For this review, take the finished solid that the model builds, in its own axes (mm). Coordinates: 2 decimals unless noted, no trailing zeros. Order: outer loops, then holes, each group sorted by start corner. A loop starts at its lowest first (then second) coordinate and runs counter-clockwise, first axis right, second up. Notation, with made-up numbers: (53.25, 77) -> (86.25, 77) arc R8 ccw to (86.25, 92) -> close; hole circle Ø8 at (8, 80.5). An arc over 180 degrees is marked (long way). Return JSON: item names as keys, results as strings. Group by question number.
Item 1: Take a section at B-B (x = -15). Write out the cut boundary in (y, z).
Item 2: For line 1 along X through (y, z) = (15.15, 10); line 2 along X through (y, z) = (15.2, 55); line 3 along Z through (x, y) = (-11, 14.8), list the stretches that pass through material, from the lowest coordinate up.
Item 3: Insertion check: pin 1 (6 mm diameter, centred on x = -2, z = 52, fed in from +Y); pin 2 (1.6 mm diameter, centred on x = -1.5, y = 11, fed in from +Z); pin 3 (1.5 mm diameter, centred on x = -0.5, z = 31.5, fed in from -Y); pin 4 (2 mm diameter, centred on x = -24, z = 12.5, fed in from -Y). Each pin has a flat end and moves straight along its axis. Give the tip position at first contact, or say it passes through.
Item 4: Take a section at D-D (x = -4). Write out the cut boundary in (y, z).
Item 5: Take a section at C-C (z = 32.5). Write out the cut boundary in (x, y).
Item 6: Take a section at A-A (z = 10). Write out the cut boundary in (x, y).
```python
from build123d import *

# Parameters (mm, degrees)
SKETCH1_W           = 45.5
SKETCH1_H           = 3
BOSS_EXTRUDE1_DEPTH = 20
SKETCH2_W           = 45.5
SKETCH2_H           = 3
BOSS_EXTRUDE2_DEPTH = 45
SKETCH3_R           = 8.25
CUT_EXTRUDE1_DEPTH  = 75.656105932
CUT_EXTRUDE2_DEPTH  = 75.656105932
BOSS_EXTRUDE4_DEPTH = 3
CUT_EXTRUDE3_DEPTH  = 75.656105932
SKETCH10_W          = 10
SKETCH10_H          = 2.5
CUT_EXTRUDE4_DEPTH  = 2
SKETCH13_W          = 3
SKETCH13_H          = 14.133974596
CUT_EXTRUDE6_DEPTH  = 1
CHAMFER1_SIZE       = 1
SKETCH15_R          = 2.25
CUT_EXTRUDE7_DEPTH  = 75.788557826
CHAMFER2_SIZE       = 1


with BuildPart() as part:
    # Sketch1 → Boss-Extrude1 (new body)
    with BuildSketch(Plane.XY):
        with Locations((-13.849646897, 14.534741944)):
            Rectangle(SKETCH1_W, SKETCH1_H)
    extrude(amount=BOSS_EXTRUDE1_DEPTH)

    # Sketch2 → Boss-Extrude2 (add)
    with BuildSketch(Plane.XY.offset(20)):
        with Locations((-13.849646897, 14.534741944)):
            Rectangle(SKETCH2_W, SKETCH2_H)
    extrude(amount=BOSS_EXTRUDE2_DEPTH)

    # Sketch3 → Cut-Extrude1 (cut, through all)
    with BuildSketch(Plane(origin=(0, 13.034741944, 0), x_dir=(-1, 0, 0), z_dir=(0, -1, 0))):
        with Locations(Location((26.924646897, -55, 0), (0, 0, 90))):
            Circle(SKETCH3_R)
        with Locations(Location((0.774646897, -55, 0), (0, 0, 90))):
            Circle(SKETCH3_R)
    extrude(amount=-CUT_EXTRUDE1_DEPTH, mode=Mode.SUBTRACT)

    # Sketch5 → Cut-Extrude2 (cut, through all)
    with BuildSketch(Plane(origin=(0, 13.034741944, 0), x_dir=(-1, 0, 0), z_dir=(0, -1, 0))):
        Polygon((29.424646897, -25), (29.424646897, -45.5), (24.424646897, -45.5), (24.424646897, -25), (25.424646897, -25), (25.424646897, -44.5), (28.424646897, -44.5), (28.424646897, -25), align=None)
        Polygon((-0.725353103, -25), (-1.725353103, -25), (-1.725353103, -45.5), (3.274646897, -45.5), (3.274646897, -25), (2.274646897, -25), (2.274646897, -44.5), (-0.725353103, -44.5), align=None)
    extrude(amount=-CUT_EXTRUDE2_DEPTH, mode=Mode.SUBTRACT)

    # Sketch6 → Boss-Extrude4 (add)
    with BuildSketch(Plane(origin=(-25.424646897, 0, 0), x_dir=(0, 0, -1), z_dir=(1, 0, 0))):
        Polygon((-44.5, 13.034741944), (-46, 12.16871654), (-46, 10.66871654), (-41.5, 10.66871654), (-39.133974596, 13.034741944), align=None)
    boss_extrude4 = extrude(amount=-BOSS_EXTRUDE4_DEPTH)

    # Mirror7: Boss-Extrude4 across plane
    add(boss_extrude4.mirror(Plane(origin=(-13.849646897, 13.034741944, 25), x_dir=(0, 0, 1), z_dir=(1, 0, 0))))

    # Sketch9 → Cut-Extrude3 (cut, through all)
    with BuildSketch(Plane(origin=(0, 13.034741944, 0), x_dir=(-1, 0, 0), z_dir=(0, -1, 0))):
        with BuildLine():
            Line((16.849646897, -65), (10.849646897, -65))
            ThreePointArc((10.849646897, -65), (8.099646897, -62.25), (10.849646897, -59.5))
            Line((10.849646897, -59.5), (16.849646897, -59.5))
            ThreePointArc((16.849646897, -59.5), (19.599646897, -62.25), (16.849646897, -65))
        make_face()
    extrude(amount=-CUT_EXTRUDE3_DEPTH, mode=Mode.SUBTRACT)

    # Sketch10 → Cut-Extrude4 (cut)
    with BuildSketch(Plane(origin=(0, 13.034741944, 0), x_dir=(-1, 0, 0), z_dir=(0, -1, 0))):
        with Locations((13.849646897, -46.25)):
            Rectangle(SKETCH10_W, SKETCH10_H)
    extrude(amount=-CUT_EXTRUDE4_DEPTH, mode=Mode.SUBTRACT)

    # Sketch13 → Cut-Extrude6 (cut)
    with BuildSketch(Plane(origin=(0, 13.034741944, 0), x_dir=(-1, 0, 0), z_dir=(0, -1, 0))):
        with Locations((26.924646897, -32.066987298)):
            Rectangle(SKETCH13_W, SKETCH13_H)
        with Locations((0.774646897, -32.066987298)):
            Rectangle(SKETCH13_W, SKETCH13_H)
    extrude(amount=-CUT_EXTRUDE6_DEPTH, mode=Mode.SUBTRACT)

    # Chamfer1
    chamfer1_edges = [part.edges().sort_by_distance(p)[0] for p in [
        (-26.924646897, 14.034741944, 25),
        (-0.774646897, 14.034741944, 25),
    ]]
    chamfer(chamfer1_edges, length=CHAMFER1_SIZE - 0.0001)  # a hair under: the kernel refuses the full size

    # Sketch15 → Cut-Extrude7 (cut, through all)
    with BuildSketch(Plane(origin=(0, 16.034741944, 0), x_dir=(1, 0, 0), z_dir=(0, 1, 0))):
        with Locations(Location((-26.599646897, -10, 0), (0, 0, 270))):
            Circle(SKETCH15_R)
        with Locations(Location((-1.099646897, -10, 0), (0, 0, 270))):
            Circle(SKETCH15_R)
    extrude(amount=-CUT_EXTRUDE7_DEPTH, mode=Mode.SUBTRACT)

    # Chamfer2
    chamfer2_edges = [part.edges().sort_by_distance(p)[0] for p in [
        (-28.424646897, 14.534791944, 25),
        (-25.424646897, 14.534791944, 25),
        (0.725353103, 14.534791944, 25),
        (-2.274646897, 14.534791944, 25),
    ]]
    chamfer(chamfer2_edges, length=CHAMFER2_SIZE - 0.0001)  # a hair under: the kernel refuses the full size


solid = part.part
```
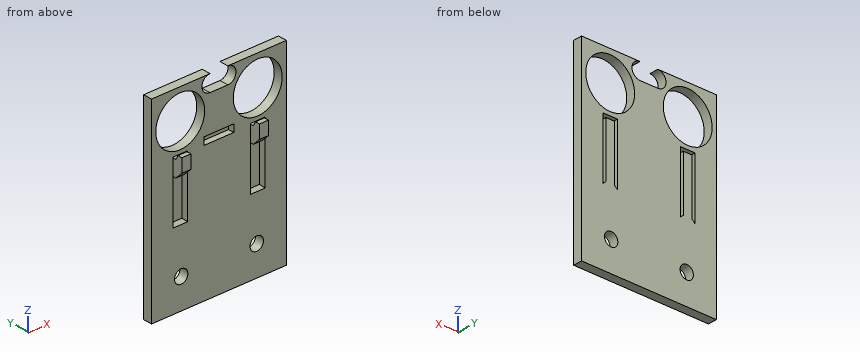
Findings below:
{
 "1": {"outline": "(13.03, 0) -> (16.03, 0) -> (16.03, 59.5) -> (13.03, 59.5) -> (13.03, 47.5) -> (15.03, 47.5) -> (15.03, 45) -> (13.03, 45) -> close"},
 "2": {"line 1": "x = -36.6 to -28.85, -24.35 to -3.35, 1.15 to 8.9", "line 2": "x = -36.6 to -35.17, -18.67 to -9.02, 7.48 to 8.9", "line 3": "z = 0 to 45, 47.5 to 59.5"},
 "3": {"pin 1": "passes through", "pin 2": "stops at z = 46", "pin 3": "stops at y = 14.03", "pin 4": "stops at y = 13.03"},
 "4": {"outline": "(13.03, 0) -> (16.03, 0) -> (16.03, 47.41) -> (13.03, 47.41) -> close; (13.03, 62.59) -> (16.03, 62.59) -> (16.03, 65) -> (13.03, 65) -> close"},
 "5": {"outline": "(-36.6, 13.03) -> (-29.42, 13.03) -> (-29.42, 16.03) -> (-36.6, 16.03) -> close; (-28.42, 14.03) -> (-25.42, 14.03) -> (-25.42, 16.03) -> (-28.42, 16.03) -> close; (-24.42, 13.03) -> (-3.27, 13.03) -> (-3.27, 16.03) -> (-24.42, 16.03) -> close; (-2.27, 14.03) -> (0.73, 14.03) -> (0.73, 16.03) -> (-2.27, 16.03) -> close; (1.73, 13.03) -> (8.9, 13.03) -> (8.9, 16.03) -> (1.73, 16.03) -> close"},
 "6": {"outline": "(-36.6, 13.03) -> (-28.85, 13.03) -> (-28.85, 16.03) -> (-36.6, 16.03) -> close; (-24.35, 13.03) -> (-3.35, 13.03) -> (-3.35, 16.03) -> (-24.35, 16.03) -> close; (1.15, 13.03) -> (8.9, 13.03) -> (8.9, 16.03) -> (1.15, 16.03) -> close"}
}
